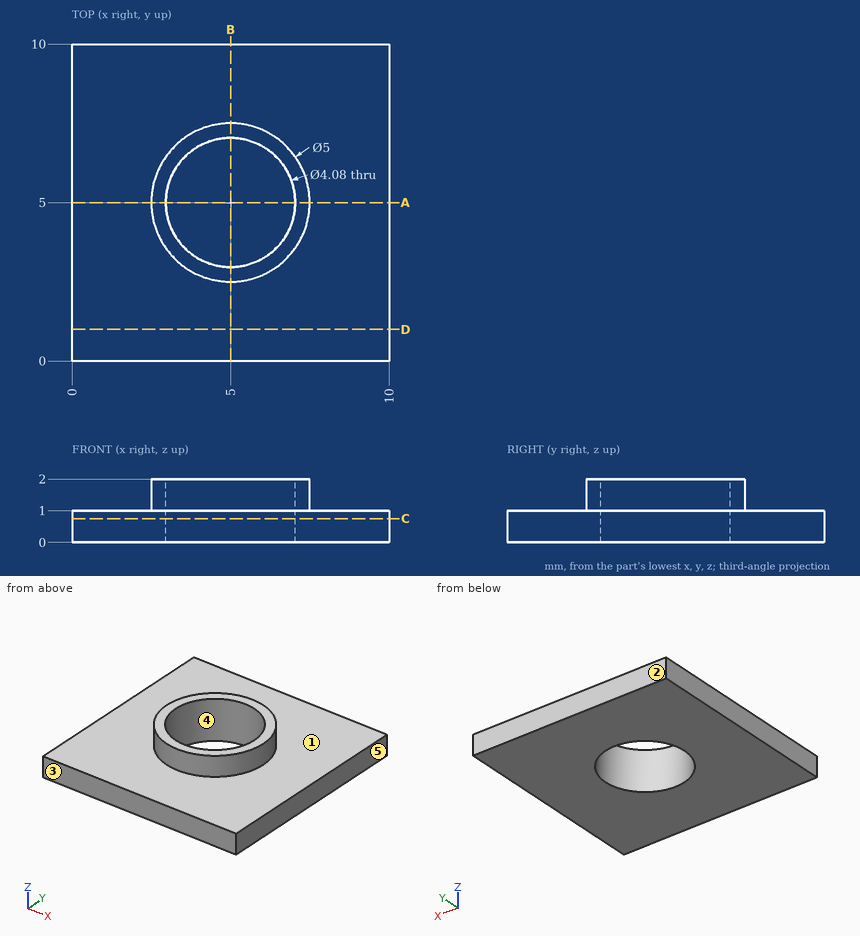
Source: three-view drawing plus pictorial views. Frame: mm from the lowest corner of the part. A direction names the side the tool comes from. Round coordinates to 2 decimals unless told otherwise and drop trailing zeros. Order: outer loops, then holes, each group sorted by start corner. A loop starts at its lowest first (then second) coordinate and runs counter-clockwise, first axis right, second up. Notation, with made-up numbers: (82.25, 73.25) -> (100.25, 73.25) arc R16 cw to (100.25, 99.25) -> close; hole circle Ø8 at (20.25, 61.5). An arc over 180 degrees is marked (long way). Use CSV: the item, a comma, the result in double quotes. Start each with the question number.
1) Set-up query: the marked faces 1 and 2. Return all of +Z, -Z, +X, -X, +Y, -Y with unobstructed straight access to the full face (end or side cutting, diameter ignored); none if empty.
2) Material intervals for line 1 along Y through (x, z) = (5, 1.1); line 2 along X through (y, z) = (5, 0.6), sorted ascending. Write a range as from..to.
3) Section A-A (y = 5). Return the cut outline in (x, z), and give its area (3 significant figures).
4) Section C-C (z = 0.75). Return the cut outline in (x, y), and give its area (3 significant figures).
5) Section D-D (y = 1). Return the cut outline in (x, z).
6) First-contact query: pin 1 Ø5.5 at (x, y) = (5, 5) entering from +Z. Flat tip, straight axial feed; report the tip coordinate or a pass-through.
7) Draft query along X for the marked faces 3, 4 and 5. Return one class per face: +X half, -X half, draft (parallel to the pull), parting line (faces both ways), or undercut.
Returned:
1,face 1,"+Z"
1,face 2,"+Z, -Z, +X, -X, +Y"
2,line 1,"y = 2.5..2.96, 7.04..7.5"
2,line 2,"x = 0..2.96, 7.04..10"
3,outline,"(0, 0) -> (2.96, 0) -> (2.96, 2) -> (2.5, 2) -> (2.5, 1) -> (0, 1) -> close; (7.04, 0) -> (10, 0) -> (10, 1) -> (7.5, 1) -> (7.5, 2) -> (7.04, 2) -> close"
3,area,"6.84 mm²"
4,outline,"(0, 0) -> (10, 0) -> (10, 10) -> (0, 10) -> close; hole circle Ø4.08 at (5, 5)"
4,area,"86.9 mm²"
5,outline,"(0, 0) -> (10, 0) -> (10, 1) -> (0, 1) -> close"
6,pin 1,"stops at z = 2"
7,face 3,"draft"
7,face 4,"undercut"
7,face 5,"+X half"
